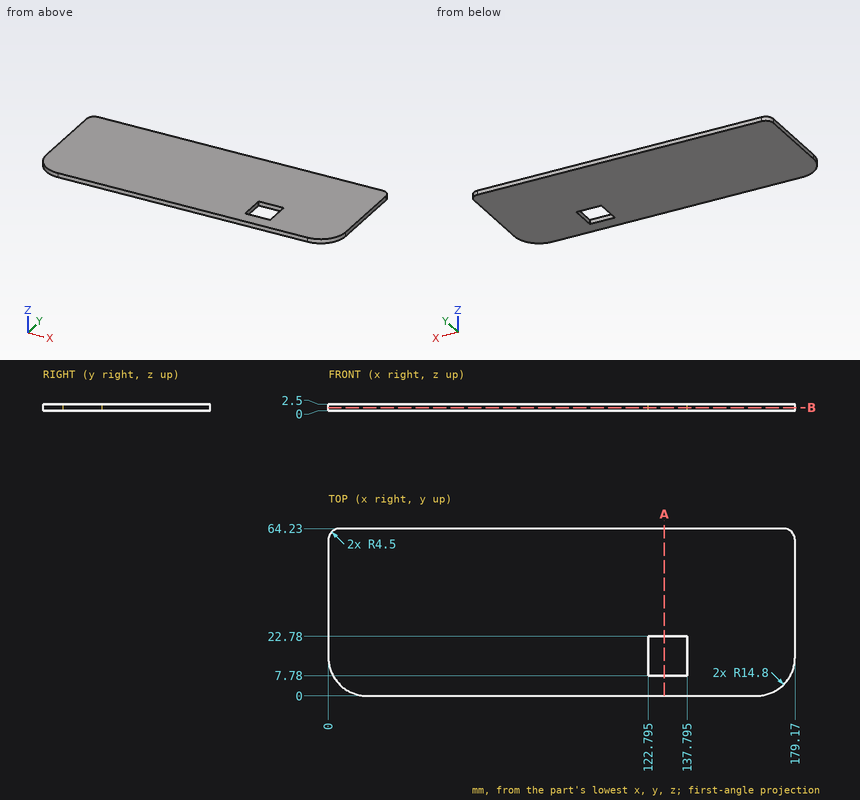
Can you work these out from the drawing? Everything is in mm from the part's minimum corner. Round coordinates to 2 decimals unless told otherwise and drop trailing zeros. Order: outer loops, then holes, each group sorted by start corner. A loop starts at its lowest first (then second) coordinate and runs counter-clockwise, first axis right, second up. Notation, with made-up numbers: M 5.5,28 L 17.5,28 A21 ccw 17.5,48 Z; hole C -22,60.5 d11. An arc over 180 degrees is marked long. One line per question, with ' | ' between items.
1) I need wall thicknesses on line 1 along Y through (x, z) = (128, 0.7); line 2 along X through (y, z) = (17.5, 0.6) (3 decimals); line 3 along X through (y, z) = (11.5, 0.7) (1 decimal). Which ranges of each line are inside material? Lowest first, please.
Working result:
line 1: 0 to 7.78, 22.78 to 64.23 | line 2: 0 to 122.795, 137.795 to 179.17 | line 3: 0.4 to 122.8, 137.8 to 178.8
2) I want a section at B-B, the plane z = 1.1. Write out the boundary of the cut face in (x, y) (3 decimals), then the cut area to 3 significant figures.
Working result:
outline: M 0,14.8 A14.8 ccw 14.8,0 L 164.37,0 A14.8 ccw 179.17,14.8 L 179.17,59.73 A4.5 ccw 174.67,64.23 L 4.5,64.23 A4.5 ccw 0,59.73 Z; hole M 122.795,7.78 L 137.795,7.78 L 137.795,22.78 L 122.795,22.78 Z | area: 11,200 mm²
3) I want a section at A-A, the plane x = 129. Write out the boundary of the cut face in (y, z), then the cut area to 3 significant figures.
Working result:
outline: M 0,0 L 7.78,0 L 7.78,2.5 L 0,2.5 Z; M 22.78,0 L 64.23,0 L 64.23,2.5 L 22.78,2.5 Z | area: 123 mm²
